Input: dimensioned drawing with shaded views. Units: mm. Origin: part minimum x, y, z. A direction names the side the tool comes from. Give positions to 0.01 mm unless a question says otherwise; leave off trailing zeros. Write each loop counter-clockwise with the first axis right and the second up, starting at its lowest first coordinate (ties: lowest second). Pieces come first, ordered by that corner, then holes. Notation, with made-up numbers: M 51.5,-30 L 58.5,-30 A24 cw 58.5,-18 Z; hole C 51,-36.75 d11. An arc over 180 degrees is marked long. Answer as a JSON object with one key per item and string values.
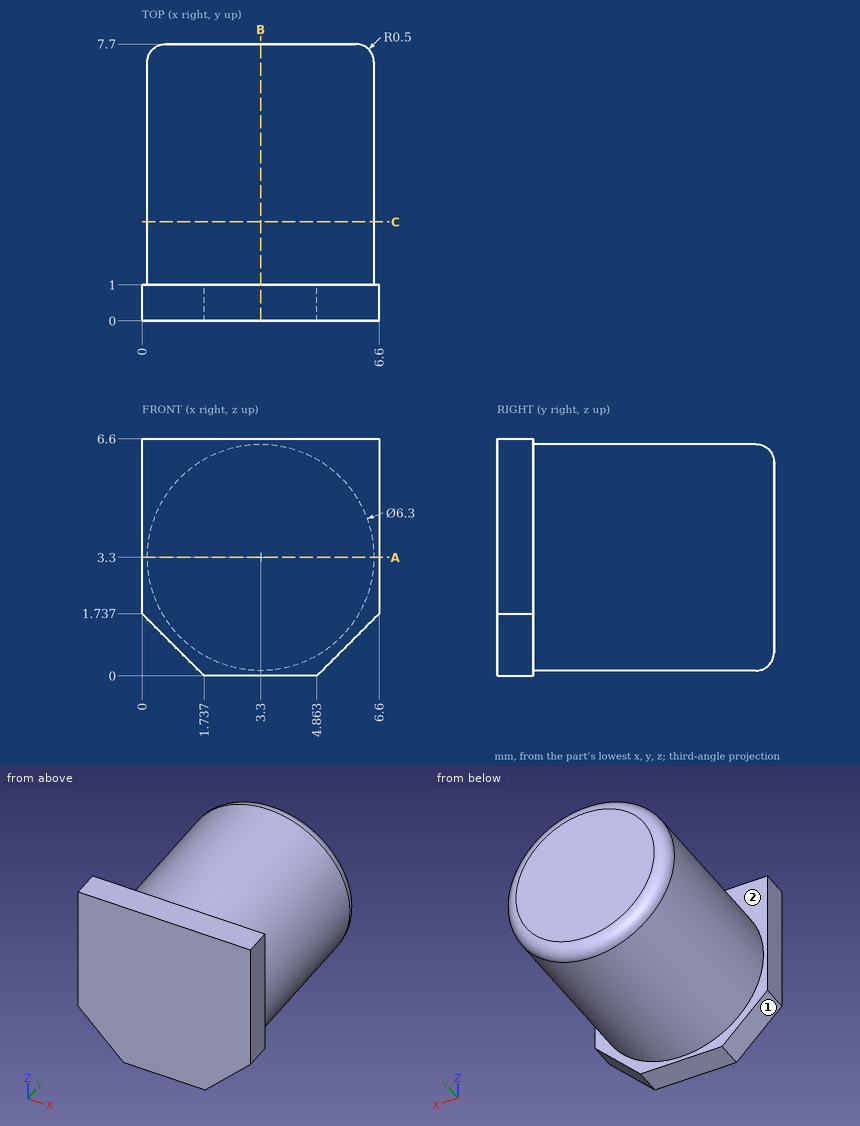
1) Line query: line 1 (Y direction, x = 6, z = 5.25); line 2 (Z direction, x = 3.25, y = 6.75); line 3 (X direction, y = 2, z = 6) (1 decimal). Output: solid intervals per line, ascending. Write a range as from..to.
Geometry check:
{"line 1": "y = 0..1", "line 2": "z = 0.15..6.45", "line 3": "x = 1.7..4.9"}
2) Set-up query: the marked faces 1 and 2. Return all of +Z, -Z, +X, -X, +Y, -Y with unobstructed straight access to the full face (end or side cutting, diameter ignored); none if empty.
Geometry check:
{"face 1": "-Z, -X, +Y, -Y", "face 2": "+Y"}
3) Cut plane A-A on z = 3.3. Return loops of the section in (x, y).
Geometry check:
{"outline": "M 0,0 L 6.6,0 L 6.6,1 L 6.45,1 L 6.45,7.2 A0.5 ccw 5.95,7.7 L 0.65,7.7 A0.5 ccw 0.15,7.2 L 0.15,1 L 0,1 Z"}
4) Cut plane C-C on y = 2.75. Return loops of the section in (x, z).
Geometry check:
{"outline": "C 3.3,3.3 d6.3"}
5) Cut plane B-B on x = 3.3. Return loops of the section in (y, z), and give its area (3 significant figures).
Geometry check:
{"outline": "M 0,0 L 1,0 L 1,0.15 L 7.2,0.15 A0.5 ccw 7.7,0.65 L 7.7,5.95 A0.5 ccw 7.2,6.45 L 1,6.45 L 1,6.6 L 0,6.6 Z", "area": "48.7 mm2"}
6) Contact query for a flat-ended pin moving along its axis: P1, Ø1.5, axis at x = 5.5, z = 3, coming from the -Y side. Output: stop coordinate, or through.
Geometry check:
{"P1": "stops at y = 0"}
